```python
from build123d import *

# Parameters (mm, degrees)
F1_DEPTH  = 16.51
F2_W      = 11.811
F2_H      = 1.5875
F3_DEPTH  = 25.909
F4_DEPTH  = 25.909
F5_R      = 3.175
F6_DEPTH  = 12.7368181024
F9_DEPTH  = 3.937
F11_DEPTH = 8.255
F12_R     = 1.016
F13_R     = 3.81
F18_DEPTH = 25.4


with BuildPart() as f1:
    # F0 (on Front) → F1 (new body)
    with BuildSketch(Plane.XZ):
        Polygon((0, 0), (15.748, 0), (15.748, 5.588), (1.3198227154, 5.588), (-6.7504579853, 19.5661362049), (-10.16, 17.5976362049), align=None)
    extrude(amount=F1_DEPTH)

    # F2 (on face) → F3 (cut, through all)
    with BuildSketch(Plane.YZ.offset(15.748)):
        with Locations((-8.255, 0.79375)):
            Rectangle(F2_W, F2_H)
    extrude(amount=-F3_DEPTH, mode=Mode.SUBTRACT)

    # F2 (on face) → F4 (cut, through all)
    with BuildSketch(Plane.YZ.offset(15.748)):
        with Locations((-8.255, 0.79375)):
            Rectangle(F2_W, F2_H)
    extrude(amount=-F4_DEPTH, mode=Mode.SUBTRACT)

    # F5 (on face) → F6 (cut, through all)
    with BuildSketch(Plane(origin=(3.4095420147, 0, 1.9685), x_dir=(0, 1, 0), z_dir=(0.8660254038, 0, 0.5))):
        with Locations((-8.255, 12.065)):
            Circle(F5_R)
    extrude(amount=-F6_DEPTH, mode=Mode.SUBTRACT)

    # F8 (on mid) → F9 (join, symmetric)
    with BuildSketch(Plane.XZ.offset(8.255)):
        Polygon((0, -2.2225), (0, 0), (-0.9165435523, 1.5875), (-1.5875, 2.749630657), (-1.5875, -6.2865), (15.748, -6.2865), (15.748, -2.2225), align=None)
    extrude(amount=F9_DEPTH, both=True)

    # F10 (on mid) → F11 (join, symmetric)
    with BuildSketch(Plane.XZ.offset(8.255)):
        Polygon((-1.5875, 0), (0, 0), (0, 1.5875), (-0.9165435523, 1.5875), (-1.5875, 2.749630657), align=None)
    extrude(amount=F11_DEPTH, both=True)

    # F12
    f12_edges = [f1.edges().sort_by_distance(p)[0] for p in [
        (-0.79375, -4.318, 0),
        (-0.79375, -12.192, 0),
    ]]
    fillet(f12_edges, radius=F12_R)

    # F13
    f13_edges = [f1.edges().sort_by_distance(p)[0] for p in [
        (-1.5875, -8.255, 2.749631),
        (1.319823, -8.255, 5.588),
    ]]
    fillet(f13_edges, radius=F13_R)

    # F15 (on mid) → F16 (revolve, cut)
    with BuildSketch(Plane.XZ.offset(8.255)):
        Polygon((9.6337636205, 4.79425), (9.6337636205, 5.588), (8.8400136205, 5.588), align=None)
    revolve(axis=Axis((9.6337636205, -8.255, 5.191125), (0, 0, -1)), mode=Mode.SUBTRACT)

    # F17 (on face) → F18 (cut)
    with BuildSketch(Plane(origin=(3.4095420147, 0, 1.9685), x_dir=(0, 1, 0), z_dir=(0.8660254038, 0, 0.5))):
        with BuildLine():
            Line((-16.51, 20.32), (-16.51, 12.065))
            ThreePointArc((-16.51, 12.065), (-14.0921664787, 17.9021664787), (-8.255, 20.32))
            Line((-8.255, 20.32), (-16.51, 20.32))
        make_face()
        with BuildLine():
            Line((0, 20.32), (-8.255, 20.32))
            ThreePointArc((-8.255, 20.32), (-2.4178335213, 17.9021664787), (0, 12.065))
            Line((0, 12.065), (0, 20.32))
        make_face()
    extrude(amount=-F18_DEPTH, mode=Mode.SUBTRACT)


solid = f1.part
```
Verification items for the finished model (mm, model axes). A direction names the side the tool comes from. Round coordinates to 2 decimals unless told otherwise and drop trailing zeros. Order: outer loops, then holes, each group sorted by start corner. A loop starts at its lowest first (then second) coordinate and runs counter-clockwise, first axis right, second up. Notation, with made-up numbers: (-27, -37.5) - (-15, -37.5) arc R17 cw to (-15, -18.5) - close; hole circle Ø8 at (33, -13). An arc over 180 degrees is marked (long way). Use CSV: the item, a comma, the result in double quotes. Start each with the question number.
1) Mould release check, pull along X, two halves, no side actions. Record for faces 5 (the flat face through (-1.588, -8, -1)), 6 (the conical face through (9.8, -8.39, 5.01)), 7 (the flat face through (7, -4.318, -4)): +X half, -X half, draft (parallel to the pull), parting line (faces both ways), or undercut.
2) Access from +Z, -Z, +X, -X, +Y, -Y to the whole of each face (thin tool, end or side, straight path). Record for faces 1 (the flat face through (7, -15, 0)), 2 (the flat face through (7, -1, 0)), 3 (the flat face through (8, -8, 1.588)), 4 (the flat face through (8, -8, -2.222)).
3) Section check C-C, the plane z = 1. Record the cut outline in (x, y).
4) Section check D-D, the plane y = -1.25. Record the cut outline in (x, z).
5) Thickness scan on L1, parallel to Z at x = 5.75, y = -6.25; L2, parallel to Y at x = 9, z = -4; L3, parallel to Z at x = 4.5, y = -2.75. Record the ranges inside material, lowest first.
6) Section check A-A, the plane x = 4.75. Record the cut outline in (y, z).
7) Go/stop test with flat-tipped pins: P1, Ø4, axis at y = -6.5, z = 16, coming from the -X side; P2, Ø8.5, axis at x = 5, y = -8.5, coming from the +Z side; P3, Ø2.5, axis at x = 8.5, y = -2, coming from the -Z side; P4, Ø8, axis at x = -3, y = -7.5, coming from the -Z side. Record where each tip stops, or that it passes through.
8) Section check B-B, the plane y = -9.5. Record the cut outline in (x, z).
Answers:
1,face 5,"-X half"
1,face 6,"undercut"
1,face 7,"draft"
2,face 1,"-Z, +X, -X, -Y"
2,face 2,"-Z, +X, -X, +Y"
2,face 3,"+X"
2,face 4,"+X, +Y, -Y"
3,outline,"(-1.59, -16.51) - (15.75, -16.51) - (15.75, -14.16) - (0, -14.16) - (0, -2.35) - (15.75, -2.35) - (15.75, 0) - (-1.59, 0) - close"
4,outline,"(-8.22, 14.23) - (-2.1, 3.63) arc R3.81 cw to (-1.59, 1.73) - (-1.59, 0) - (15.75, 0) - (15.75, 5.59) - (3.52, 5.59) arc R3.81 cw to (0.22, 7.49) - (-4.81, 16.2) - close"
5,L1,"z = -6.29 to -2.22, 1.59 to 5.59"
5,L2,"y = -12.19 to -4.32"
5,L3,"z = 1.59 to 5.59"
6,outline,"(-16.51, 0) - (-14.16, 0) - (-14.16, 1.59) - (-2.35, 1.59) - (-2.35, 0) - (0, 0) - (0, 5.59) - (-16.51, 5.59) - close; (-12.19, -6.29) - (-4.32, -6.29) - (-4.32, -2.22) - (-12.19, -2.22) - close"
7,P1,"stops at x = -10.15"
7,P2,"stops at z = 6.78"
7,P3,"stops at z = 0"
7,P4,"stops at z = -6.29"
8,outline,"(-10.11, 17.52) - (-7.49, 12.98) - (-4.08, 14.95) - (-6.7, 19.48) - close; (-4.57, 7.92) - (-2.1, 3.63) arc R3.81 cw to (-1.59, 1.73) - (-1.59, -6.29) - (15.75, -6.29) - (15.75, -2.22) - (0, -2.22) - (0, 1.59) - (15.75, 1.59) - (15.75, 5.59) - (3.52, 5.59) arc R3.81 cw to (0.22, 7.49) - (-1.16, 9.89) - close"
